```python
from build123d import *

# Parameters (mm, degrees)
F0_R          = 12.7
F1_DEPTH      = 101.6
F2_T          = -9.525
F3_W          = 8.89
F3_H          = 91.44
F4_DEPTH      = 12.701
F4_DEPTH_BACK = 25.4
F5_R          = 6.35
F6_DEPTH      = 25.4
F7_R          = 4.445
F8_DEPTH      = 25.4


# Not quite as in the source:
# - a length typed as a fraction of an inch, garbled in the dataset ("3 / 203.2 mm" for 3/8 in), is restored


with BuildPart() as f1:
    # F0 (on Top) → F1 (new body)
    with BuildSketch(Plane.XY):
        Circle(F0_R)
    extrude(amount=F1_DEPTH)

    # F2 (hollow: no face is removed)
    offset(amount=F2_T, mode=Mode.SUBTRACT)

    # F3 (on Front) → F4 (cut, two sides)
    with BuildSketch(Plane.XZ) as f4_sk:
        with Locations((-4.445, 50.8)):
            Rectangle(F3_W, F3_H)
        with Locations((4.445, 50.8)):
            Rectangle(F3_W, F3_H)
    extrude(amount=-F4_DEPTH, mode=Mode.SUBTRACT)
    extrude(f4_sk.sketch, amount=F4_DEPTH_BACK, mode=Mode.SUBTRACT)

    # F5 (on face) → F6 (cut)
    with BuildSketch(Plane.XY.offset(101.6)):
        Circle(F5_R)
    extrude(amount=-F6_DEPTH, mode=Mode.SUBTRACT)

    # F7 (on face) → F8 (cut)
    with BuildSketch(Plane.XY.offset(5.08)):
        Circle(F7_R)
    extrude(amount=-F8_DEPTH, mode=Mode.SUBTRACT)


solid = f1.part
```
The listing builds one solid part. Answer for the finished solid, in the listing's coordinates (mm). A direction names the side the tool comes from. Coordinates: 2 decimals unless noted, no trailing zeros. Write each loop counter-clockwise with the first axis right and the second up, starting at its lowest first coordinate (ties: lowest second). Pieces come first, ordered by that corner, then holes. Notation, with made-up numbers: (-7, -39) - (8, -39) arc R29 ccw to (8, -6) - close; hole circle Ø5 at (54.5, -34.75). An arc over 180 degrees is marked (long way). Return JSON: item names as keys, results as strings. Group by question number.
1. A cutting plane is placed at C-C, the plane z = 11. Determine the outline of the cut face in (x, y), plus the area to 3 significant figures.
2. A cutting plane is placed at A-A, the plane y = 0. Determine the outline of the cut face in (x, z) (3 decimals), plus the area to 3 significant figures.
3. A cutting plane is placed at D-D, the plane x = -7.75. Determine the outline of the cut face in (y, z), plus the area to 3 significant figures.
4. Determine the mould class of faces 4 (the flat face through (3, 6, 101.6)), 5 (the flat face through (8.89, 0, 50)), 6 (the cylindrical face through (-0.96, -4.34, 2.58)) for opening direction Z: released by +Z, released by -Z, zero draft, split by the parting line, or undercut.
5. Given pin 1 (2 mm diameter, centred on y = -10, z = 63.5, fed in from -X); pin 2 (1.5 mm diameter, centred on y = 9.5, z = 16.5, fed in from +X); pin 3 (3 mm diameter, centred on y = -5.5, z = 81.5, fed in from -X), each flat-ended and moving along its own axis, determine where each tip first touches the part or whether it passes through.
6. A cutting plane is placed at B-B, the plane x = 0. Determine the outline of the cut face in (y, z) (3 decimals), plus the area to 3 significant figures.
7. Which of the six approach directions +Z, -Z, +X, -X, +Y, -Y give full straight-line access (tool end or side, diameter ignored) to faces 1 (the flat face through (-8.89, 0, 50)), 2 (the cylindrical face through (-1.38, -6.2, 99.1)), 3 (the flat face through (5, 0, 0))?
8. Straight lines are drawn through the part: L1, parallel to Z at x = -6.5, y = 2.25; L2, parallel to Y at x = 0, z = 3.6 (3 decimals); L3, parallel to Z at x = -4, y = 2.5. For each, find the intervals that lie inside material, in ascending order.
Ans:
{
 "1": {"outline": "(-8.89, -9.07) - (-8.89, 9.07) arc R12.7 ccw to start; (8.89, -9.07) arc R12.7 ccw to (8.89, 9.07) - close", "area": "95.3 mm²"},
 "2": {"outline": "(-12.7, 0) - (-4.445, 0) - (-4.445, 5.08) - (-8.89, 5.08) - (-8.89, 96.52) - (-6.35, 96.52) - (-6.35, 101.6) - (-12.7, 101.6) - close; (4.445, 0) - (12.7, 0) - (12.7, 101.6) - (6.35, 101.6) - (6.35, 96.52) - (8.89, 96.52) - (8.89, 5.08) - (4.445, 5.08) - close", "area": "845 mm²"},
 "3": {"outline": "(-10.06, 0) - (10.06, 0) - (10.06, 5.08) - (-10.06, 5.08) - close; (-10.06, 96.52) - (10.06, 96.52) - (10.06, 101.6) - (-10.06, 101.6) - close", "area": "204 mm²"},
 "4": {"face 4": "released by +Z", "face 5": "undercut", "face 6": "zero draft"},
 "5": {"pin 1": "x = -8.96", "pin 2": "x = 9.2", "pin 3": "x = -12.05"},
 "6": {"outline": "(-12.7, 0) - (-4.445, 0) - (-4.445, 5.08) - (-12.7, 5.08) - close; (-12.7, 96.52) - (-6.35, 96.52) - (-6.35, 101.6) - (-12.7, 101.6) - close; (4.445, 0) - (12.7, 0) - (12.7, 5.08) - (4.445, 5.08) - close; (6.35, 96.52) - (12.7, 96.52) - (12.7, 101.6) - (6.35, 101.6) - close", "area": "148 mm²"},
 "7": {"face 1": "+Y, -Y", "face 2": "+Z", "face 3": "-Z, +X, -X, +Y, -Y"},
 "8": {"L1": "0 to 5.08, 96.52 to 101.6", "L2": "-12.7 to -4.445, 4.445 to 12.7", "L3": "0 to 5.08"}
}
